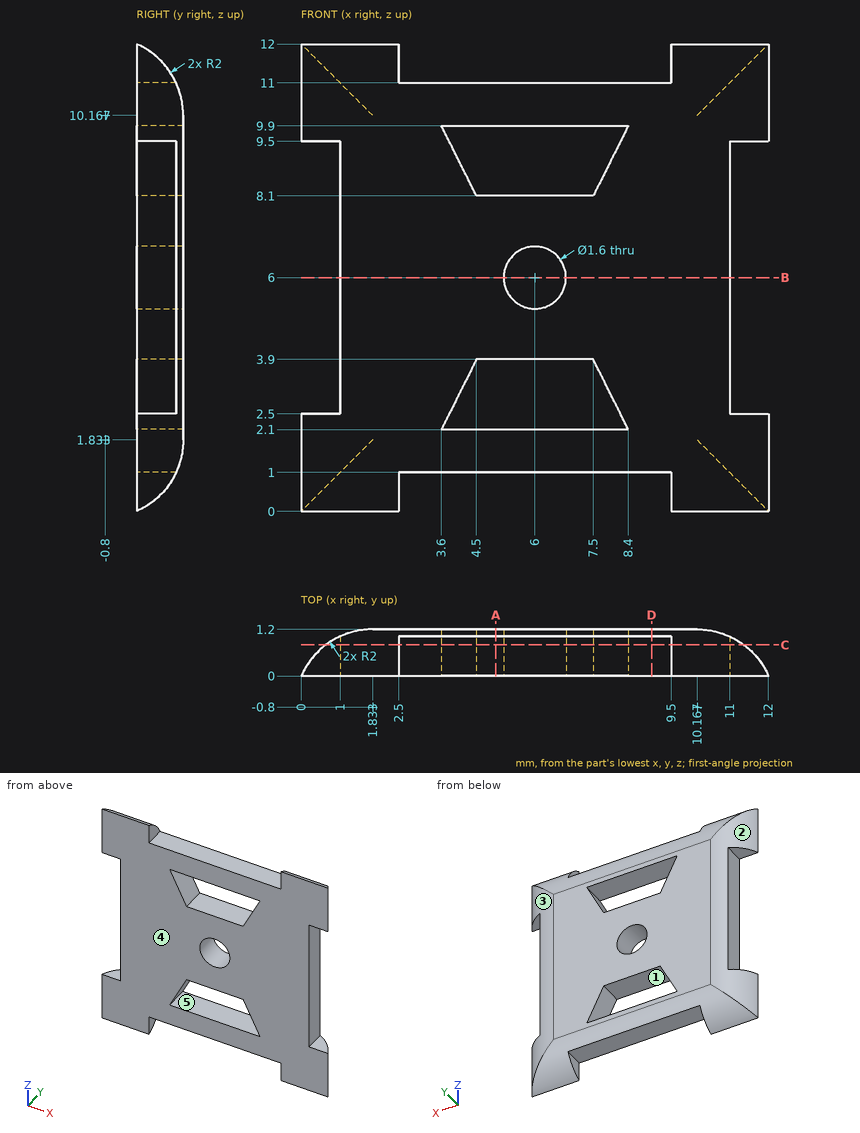
Print and shaded views of the part. All mm, measured from the part's lowest x, y and z. A direction names the side the tool comes from. Give positions to 0.01 mm unless a question says otherwise; leave off trailing zeros. Order: outer loops, then holes, each group sorted by start corner. A loop starts at its lowest first (then second) coordinate and runs counter-clockwise, first axis right, second up. Notation, with made-up numbers: (-32, 39.25) - (-21, 39.25) arc R14 cw to (-21, 46.25) - close; hole circle Ø9 at (-24, -23). An arc over 180 degrees is marked (long way). One line per item, written item: value.
Item 1: Slice it at A-A (x = 5). List the corners of the cut face in (y, z), then the cut area to 3 significant figures.
Response values:
outline: (0, 1) - (1.02, 1) arc R2 ccw to (1.2, 1.83) - (1.2, 2.1) - (0, 2.1) - close; (0, 3.9) - (1.2, 3.9) - (1.2, 8.1) - (0, 8.1) - close; (0, 9.9) - (1.2, 9.9) - (1.2, 10.17) arc R2 ccw to (1.02, 11) - (0, 11) - close
area: 7.58 mm2
Item 2: Slice it at C-C (y = 0.8). Give the number of separate pieces and of enclosed holes in the cut face, then the cut area to 3 significant figures.
Response values:
separate pieces: 1
enclosed holes: 3
area: 88.9 mm2
Item 3: Two-plate mould, pull along X, no slides. Class the marked faces 1, 2 and 3: released by +X, released by -X, zero draft, split by the parting line, or undercut.
Response values:
face 1: undercut
face 2: released by -X
face 3: released by +X
Item 4: Wall check: line 1 (Z direction, x = 6, y = 0.6); line 2 (X direction, y = 0.5, z = 6); line 3 (X direction, y = 0.2, z = 8). Give the ranges that are in metal, low to high.
Response values:
line 1: 1 to 2.1, 3.9 to 5.2, 6.8 to 8.1, 9.9 to 11
line 2: 1 to 5.2, 6.8 to 11
line 3: 1 to 11
Item 5: Tool access for the marked faces 4 and 5: list every direction of +Z, -Z, +X, -X, +Y, -Y with a clear straight run to the whole face (end or side of a thin tool).
Response values:
face 4: +Z, -Z, +X, -X, -Y
face 5: +Y, -Y
Item 6: Slice it at D-D (x = 9). List the corners of the cut face in (y, z), then the cut area to 3 significant figures.
Response values:
outline: (0, 1) - (1.02, 1) arc R2 ccw to (1.2, 1.83) - (1.2, 10.17) arc R2 ccw to (1.02, 11) - (0, 11) - close
area: 11.9 mm2
Item 7: Slice it at B-B (z = 6). List the corners of the cut face in (x, y), then the cut area to 3 significant figures.
Response values:
outline: (1, 0) - (5.2, 0) - (5.2, 1.2) - (1.83, 1.2) arc R2 ccw to (1, 1.02) - close; (6.8, 0) - (11, 0) - (11, 1.02) arc R2 ccw to (10.17, 1.2) - (6.8, 1.2) - close
area: 9.98 mm2
Item 8: Pin check, flat tips, straight feed: pin 1 Ø0.5 at (x, y) = (11.5, 0.5) entering from +Z; pin 2 Ø0.6 at (x, y) = (6.5, 0.5) entering from -Z; pin 3 Ø0.5 at (y, z) = (0.5, 0.5) entering from -X. Stop position of each tip, or through.
Response values:
pin 1: z = 11.87
pin 2: z = 1
pin 3: x = 0.13
